Can you work these out from the model? Positions are in its coordinate system, mm. Give positions to 0.01 mm unless a question says otherwise; leave off trailing zeros. Loops run counter-clockwise (first coordinate to the right, second up) from the corner with the lowest first, then second, coordinate; pieces in that order, holes last. Notation, with made-up numbers: M 57.5,59.5 L 67.5,59.5 A32 cw 67.5,93.5 Z; hole C 67,-34.5 d3. An arc over 180 degrees is marked long. Use CSV: the item, a comma, the result in double quotes.
from build123d import *

# Parameters (mm, degrees)
SKETCH1_R           = 12.7
BOSS_EXTRUDE1_DEPTH = 3.175


with BuildPart() as part:
    # Sketch1 → Boss-Extrude1 (new body)
    with BuildSketch(Plane.XY):
        with BuildLine():
            add(Edge.make_bspline(
                [(1180.257267692, 35.008813197), (1193.139660075, 40.367726318), (1206.502168928, 44.757651465), (1220.202331731, 48.102785241), (1234.110916593, 50.369156642), (1248.066405738, 51.549120089)],
                knots=[0, 0, 0, 0, 0, 0, 1, 1, 1, 1, 1, 1], degree=5, weights=[1, 1, 1, 1, 1, 1]))
            add(Edge.make_bspline(
                [(1248.066405738, 51.549120089), (1265.679828886, 52.474823917), (1283.368004198, 52.789080637), (1301.370484818, 52.480125285), (1319.15681764, 51.563533118), (1336.889341522, 50.02497466)],
                knots=[0, 0, 0, 0, 0, 0, 1, 1, 1, 1, 1, 1], degree=5, weights=[1, 1, 1, 1, 1, 1]))
            Line((1336.889341522, 50.02497466), (1752.808980038, 13.93780041))
            Line((1752.808980038, 13.93780041), (1754.345072535, 13.803055131))
            add(Edge.make_bspline(
                [(1754.345072535, 13.803055131), (1758.163986963, 13.377520973), (1761.808331334, 11.637779034), (1764.656991405, 8.697593334), (1767.912340295, 1.401754935), (1766.036876744, -6.330059827), (1763.761554618, -9.699687787), (1760.566866313, -12.006562455), (1757.008478216, -13.102648357)],
                knots=[0, 0, 0, 0, 0, 0, 0.499136526, 0.499136526, 0.499136526, 1, 1, 1, 1, 1, 1], degree=5, weights=[1, 1, 1, 1, 1, 1, 1, 1, 1]))
            add(Edge.make_bspline(
                [(1757.008478216, -13.102648357), (1755.921130701, -13.437582626), (1754.801749829, -13.705134636), (1753.693337404, -13.893612086), (1752.554243561, -14.012542135), (1751.412280363, -14.061025297)],
                knots=[0, 0, 0, 0, 0, 0, 1, 1, 1, 1, 1, 1], degree=5, weights=[1, 1, 1, 1, 1, 1]))
            Line((1751.412280363, -14.061025297), (1244.434737181, -35.48015746))
            add(Edge.make_bspline(
                [(1244.434737181, -35.48015746), (1237.20914689, -35.785429122), (1229.977046286, -35.935307578), (1222.765615669, -35.931234225), (1215.551331729, -35.772585361), (1208.350739251, -35.45985118)],
                knots=[2.45e-07, 2.45e-07, 2.45e-07, 2.45e-07, 2.45e-07, 2.45e-07, 1, 1, 1, 1, 1, 1], degree=5, weights=[1, 1, 1, 1, 1, 1]))
            add(Edge.make_bspline(
                [(1208.350739251, -35.45985118), (1202.466477316, -35.112672095), (1196.591377285, -34.427059535), (1190.765084976, -33.40383537), (1185.022373471, -32.050408368), (1179.399562393, -30.382176523)],
                knots=[0, 0, 0, 0, 0, 0, 1, 1, 1, 1, 1, 1], degree=5, weights=[1, 1, 1, 1, 1, 1]))
            add(Edge.make_bspline(
                [(1179.399562393, -30.382176523), (1176.308617194, -29.465123967), (1173.297136008, -28.243926124), (1170.408947138, -26.729193922), (1167.683819714, -24.940258655), (1165.157103336, -22.905582819)],
                knots=[0, 0, 0, 0, 0, 0, 1, 1, 1, 1, 1, 1], degree=5, weights=[1, 1, 1, 1, 1, 1]))
            add(Edge.make_bspline(
                [(1165.157103336, -22.905582819), (1158.48797036, -17.53516411), (1153.722824671, -9.797202261), (1152.048165632, -0.661270673), (1153.715186732, 8.163030967), (1157.908663687, 15.423698563)],
                knots=[0, 0, 0, 0, 0, 0, 1, 1, 1, 1, 1, 1], degree=5, weights=[1, 1, 1, 1, 1, 1]))
            add(Edge.make_bspline(
                [(1157.908663687, 15.423698563), (1160.887782958, 20.581804011), (1164.761606365, 25.336166686), (1169.428635805, 29.436314437), (1174.678948991, 32.688303087), (1180.257267692, 35.008813197)],
                knots=[0, 0, 0, 0, 0, 0, 1, 1, 1, 1, 1, 1], degree=5, weights=[1, 1, 1, 1, 1, 1]))
        make_face()
        with Locations((1397, 0)):
            Circle(SKETCH1_R, mode=Mode.SUBTRACT)
        with Locations((1219.2, 0)):
            Circle(SKETCH1_R, mode=Mode.SUBTRACT)
    extrude(amount=BOSS_EXTRUDE1_DEPTH)


solid = part.part
Q1. If we mould it in two halves opening along X, with no side actions, what happens to faces 1 (the flat face through (1396, 19, 0)), 2 (the cylindrical face through (1209.1, -7.7, 1.6)), 3 (the cylindrical face through (1409.114, 3.815, 1.565)), 4 (the flat face through (1501.47, -24.62, 1.57))? For each: released by +X, released by -X, zero draft, split by the parting line, or undercut.
Model answer:
face 1,"zero draft"
face 2,"undercut"
face 3,"undercut"
face 4,"released by +X"
Q2. I want a section at A-A, the plane x = 1397. Please give me the cut outline in (y, z) (3 decimals).
Model answer:
outline,"M -29.034,0 L -12.7,0 L -12.7,3.175 L -29.034,3.175 Z; M 12.7,0 L 44.809,0 L 44.809,3.175 L 12.7,3.175 Z"
Q3. I want a section at B-B, the plane y = 0. State how many separate pieces and enclosed holes the cut face has, then the cut area to 3 significant figures.
Model answer:
separate pieces,"3"
enclosed holes,"0"
area,"1,780 mm2"
Q4. I want a section at C-C, the plane x = 1543.5. Please give me the cut outline in (y, z) (3 decimals).
Model answer:
outline,"M -22.845,0 L 32.098,0 L 32.098,3.175 L -22.845,3.175 Z"
Q5. I'm going to push a flat-ended pin straight in: P1, Ø2, axis at x = 1474, y = 27.5, coming from the -Z side. Where does the tip first touch, or does it pass through?
Model answer:
P1,"z = 0"
Q6. Please list where these lines run through material, in increasing order: L1, parallel to X at y = -9.5, z = 1; L2, parallel to Y at x = 1397, z = 1.8; L3, parallel to X at y = 4, z = 0.35. Write a range as from..to.
Model answer:
L1,"1155.65..1210.77, 1227.63..1388.57, 1405.43..1762.85"
L2,"-29.03..-12.7, 12.7..44.81"
L3,"1154.13..1207.15, 1231.25..1384.95, 1409.05..1766.11"
